Geometry check sheet. Reference: the model listing, model coordinates, mm. A direction names the side the tool comes from. Round coordinates to 2 decimals unless told otherwise and drop trailing zeros. Write each loop counter-clockwise with the first axis right and the second up, starting at its lowest first coordinate (ties: lowest second). Pieces come first, ordered by that corner, then holes.
Item 1: Cross-section at A-A (x = 35). Enter the section's corners in (y, z), then the cut area to 3 significant figures.
Item 2: Cross-section at B-B (z = 130). Enter the section's corners in (x, y), then the cut area to 3 significant figures.
Item 3: Draft check along X on faces 1 (the face through (-30.54, 8.62, 129.41)), 2 (the face through (45, 12, 99)), 3 (the face through (-41, 3, 99)), 4 (the face through (1, 0, 99)). Enter one of: pulls with the +X half, pulls with the -X half, needs draft (parallel to the pull), parting line crosses it, or undercut.
Item 4: Scan lines: probe 1 along X at (y, z) = (8.5, 70); probe 2 along Z at (x, y) = (-35, 10.5); probe 3 along X at (y, z) = (14.5, 20.5). Record each from-to range of solid material in increasing order.
Item 5: Cross-section at D-D (x = -21.5). Enter the section's corners in (y, z), then the cut area to 3 significant figures.
Item 6: Cross-section at C-C (z = 82). Enter the section's corners in (x, y), then the cut area to 3 significant figures.
Item 7: Access from +Z, -Z, +X, -X, +Y, -Y to the whole of each face (thin tool, end or side, straight path). Record for faces 5 (the face through (-25, 15, 99)), 6 (the face through (31.01, 8.62, 72.08)).
Item 8: Depth check by flat-ended pin: P1, Ø8, axis at x = -23.5, z = 110, coming from the +Y side; P2, Ø1.5, axis at x = -17, z = 111.5, coming from the +Y side; P3, Ø5.5, axis at x = 35, z = 70, coming from the -Y side. Enter the tip coordinate at first touch or a pass-through.
from build123d import *

# Parameters (mm, degrees)
EXTRUDE_1_DEPTH             = 200
CUT_EXTRUDE_1_REACH         = 207.704
SKETCH_2_R                  = 4.5
PATTERN_LINEAR_1_COUNT      = 2
PATTERN_LINEAR_1_PITCH      = 60
PATTERN_LINEAR_1_COUNT_DIR2 = 2
PATTERN_LINEAR_1_PITCH_DIR2 = 70


with BuildPart() as part:
    # 草图1 → 凸台-拉伸1 (new body)
    with BuildSketch(Plane.XY):
        Polygon((38, 0), (-38, 0), (-45, 7), (-45, 17), (-25, 17), (-25, 12), (25, 12), (25, 17), (45, 17), (45, 7), align=None)
    extrude(amount=EXTRUDE_1_DEPTH)

    # 草图2 → 切除-拉伸1 (cut, up to next)
    with BuildSketch(Plane(origin=(0, 17, 0), x_dir=(1, 0, 0), z_dir=(0, 1, 0)), mode=Mode.PRIVATE) as cut_extrude_1_sk1:
        with Locations(Location((-35, -130, 0), (0, 0, 270))):
            Circle(SKETCH_2_R)
    cut_extrude_1_tool1 = extrude(cut_extrude_1_sk1.sketch, amount=-CUT_EXTRUDE_1_REACH, mode=Mode.PRIVATE) & part.part
    cut_extrude_1 = cut_extrude_1_tool1.solids().sort_by_distance((-35, 17, 130))[0]
    add(cut_extrude_1, mode=Mode.SUBTRACT)

    # 阵列(线性)1: 切除-拉伸1; each copy of 切除-拉伸1 runs up to whatever stops it at its own place
    pattern_linear_1_before = part.part  # the part as the pattern finds it: every copy runs up to it
    pattern_linear_1_cut_extrude_1_long = extrude(cut_extrude_1_sk1.sketch, amount=-CUT_EXTRUDE_1_REACH, mode=Mode.PRIVATE)
    pattern_linear_1_cut_extrude_1_tool1 = pattern_linear_1_cut_extrude_1_long.moved(Location(Vector(0, 0, -1) * (0 * PATTERN_LINEAR_1_PITCH) + Vector(1, 0, 0) * (1 * PATTERN_LINEAR_1_PITCH_DIR2))) & pattern_linear_1_before
    add(pattern_linear_1_cut_extrude_1_tool1.solids().sort_by_distance((35, 17, 130))[0], mode=Mode.SUBTRACT)
    pattern_linear_1_cut_extrude_1_tool2 = pattern_linear_1_cut_extrude_1_long.moved(Location(Vector(0, 0, -1) * (1 * PATTERN_LINEAR_1_PITCH) + Vector(1, 0, 0) * (0 * PATTERN_LINEAR_1_PITCH_DIR2))) & pattern_linear_1_before
    add(pattern_linear_1_cut_extrude_1_tool2.solids().sort_by_distance((-35, 17, 70))[0], mode=Mode.SUBTRACT)
    pattern_linear_1_cut_extrude_1_tool3 = pattern_linear_1_cut_extrude_1_long.moved(Location(Vector(0, 0, -1) * (1 * PATTERN_LINEAR_1_PITCH) + Vector(1, 0, 0) * (1 * PATTERN_LINEAR_1_PITCH_DIR2))) & pattern_linear_1_before
    add(pattern_linear_1_cut_extrude_1_tool3.solids().sort_by_distance((35, 17, 70))[0], mode=Mode.SUBTRACT)


solid = part.part
Resolved:
1. outline: (0, 0) - (17, 0) - (17, 65.5) - (0, 65.5) - close; (0, 74.5) - (17, 74.5) - (17, 125.5) - (0, 125.5) - close; (0, 134.5) - (17, 134.5) - (17, 200) - (0, 200) - close
1. area: 3,090 mm2
2. outline: (-45, 7) - (-39.5, 1.5) - (-39.5, 17) - (-45, 17) - close; (-30.5, 0) - (30.5, 0) - (30.5, 17) - (25, 17) - (25, 12) - (-25, 12) - (-25, 17) - (-30.5, 17) - close; (39.5, 1.5) - (45, 7) - (45, 17) - (39.5, 17) - close
2. area: 927 mm2
3. face 1: undercut
3. face 2: pulls with the +X half
3. face 3: pulls with the -X half
3. face 4: needs draft
4. probe 1: x = -45 to -39.5, -30.5 to 30.5, 39.5 to 45
4. probe 2: z = 0 to 65.5, 74.5 to 125.5, 134.5 to 200
4. probe 3: x = -45 to -25, 25 to 45
5. outline: (0, 0) - (12, 0) - (12, 200) - (0, 200) - close
5. area: 2,400 mm2
6. outline: (-45, 7) - (-38, 0) - (38, 0) - (45, 7) - (45, 17) - (25, 17) - (25, 12) - (-25, 12) - (-25, 17) - (-45, 17) - close
6. area: 1,230 mm2
7. face 5: +Z, -Z, +Y
7. face 6: +Y, -Y
8. P1: stops at y = 17
8. P2: stops at y = 12
8. P3: passes through
